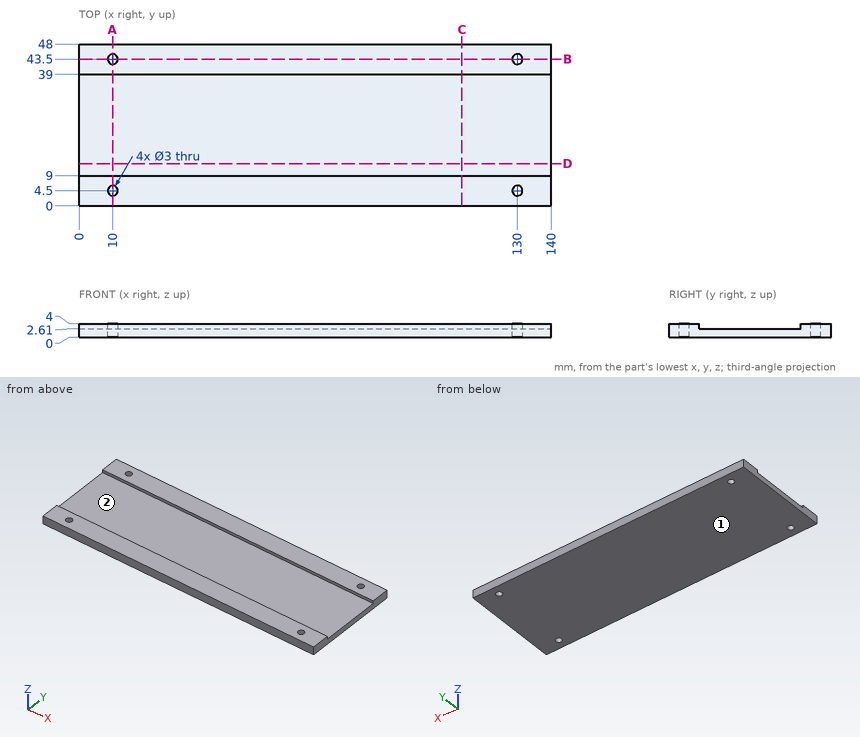
Source: three-view drawing plus pictorial views. Frame: mm from the lowest corner of the part. Give positions to 0.01 mm unless a question says otherwise; leave off trailing zeros. Order: outer loops, then holes, each group sorted by start corner. A loop starts at its lowest first (then second) coordinate and runs counter-clockwise, first axis right, second up. Notation, with made-up numbers: M -10.75,-20 L 5.25,-20 A23 ccw 5.25,-7 Z; hole C 72.5,49 d11. An arc over 180 degrees is marked long. Return JSON: item names as keys, results as strings.
Item 1: Cut plane D-D (y = 12.5). Return loops of the section in (x, z), then the cut area to 3 significant figures.
Solutions:
{"outline": "M 0,0 L 140,0 L 140,2.61 L 0,2.61 Z", "area": "365 mm^2"}
Item 2: Cut plane B-B (y = 43.5). Return loops of the section in (x, z).
Solutions:
{"outline": "M 0,0 L 8.5,0 L 8.5,4 L 0,4 Z; M 11.5,0 L 128.5,0 L 128.5,4 L 11.5,4 Z; M 131.5,0 L 140,0 L 140,4 L 131.5,4 Z"}
Item 3: First-contact query: P1, Ø10, axis at x = 55.5, y = 36, coming from the +Z side; P2, Ø8, axis at x = 79.5, y = 33.5, coming from the +Z side; P3, Ø2.5, axis at x = 10, y = 43.5, coming from the -Z side (3 decimals). Flat tips, straight axial feed; report the tip coordinate or a pass-through.
Solutions:
{"P1": "z = 4", "P2": "z = 2.61", "P3": "through"}
Item 4: Pull-direction query (Y, two-part tool) for the marked faces 1 and 2; classes: +Y half, -Y half, draft (parallel to the pull), parting line (faces both ways), or undercut.
Solutions:
{"face 1": "draft", "face 2": "undercut"}
Item 5: Cut plane A-A (x = 10). Return loops of the section in (y, z).
Solutions:
{"outline": "M 0,0 L 3,0 L 3,4 L 0,4 Z; M 6,0 L 42,0 L 42,4 L 39,4 L 39,2.61 L 9,2.61 L 9,4 L 6,4 Z; M 45,0 L 48,0 L 48,4 L 45,4 Z"}
Item 6: Cut plane C-C (x = 113.5). Return loops of the section in (y, z).
Solutions:
{"outline": "M 0,0 L 48,0 L 48,4 L 39,4 L 39,2.61 L 9,2.61 L 9,4 L 0,4 Z"}
Item 7: Ray query, probe 1 along Y at (x, z) = (130, 2.8); probe 2 along Y at (x, z) = (10, 1.4); probe 3 along Y at (x, z) = (95.5, 3.3). Return the intervals inside material, ascending.
Solutions:
{"probe 1": "0 to 3, 6 to 9, 39 to 42, 45 to 48", "probe 2": "0 to 3, 6 to 42, 45 to 48", "probe 3": "0 to 9, 39 to 48"}
